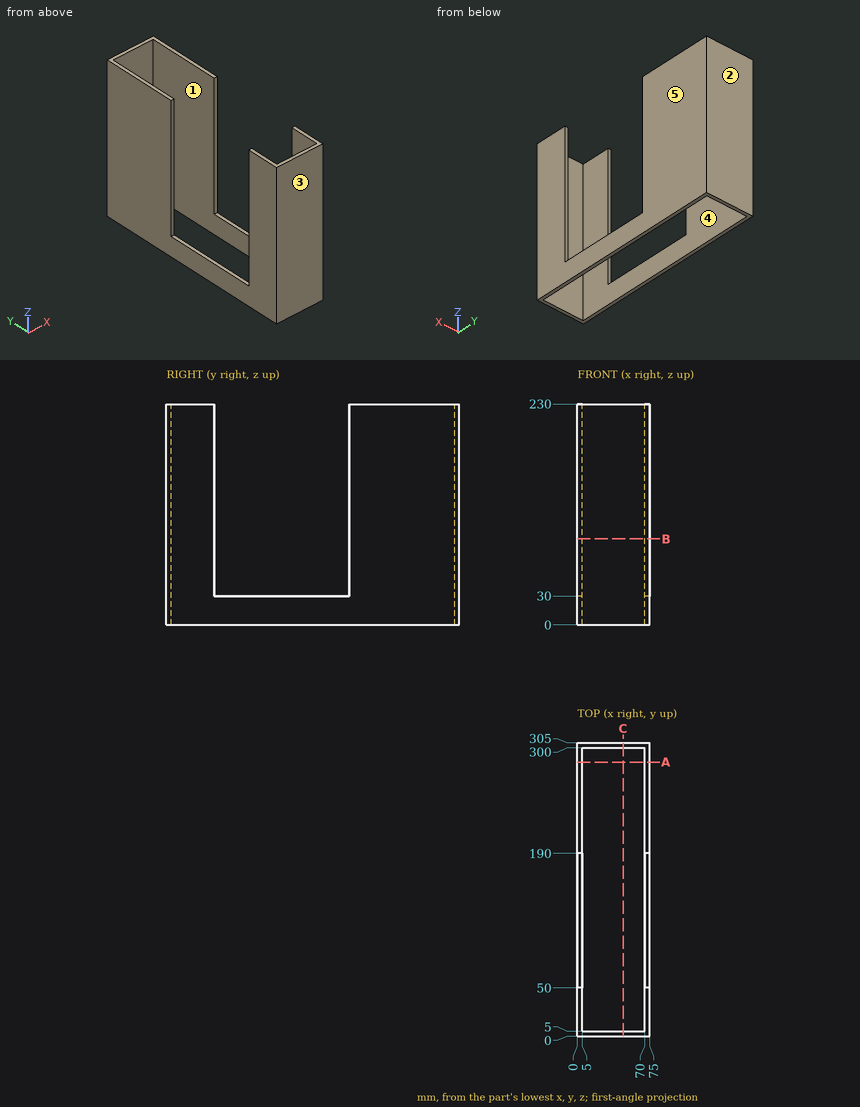
Study the drawing (mm; zero at the part's minimum x, y, z) and answer. A direction names the side the tool comes from. Coordinates: 2 decimals unless noted, no trailing zeros. Loops run counter-clockwise (first coordinate to the right, second up) from the corner with the lowest first, then second, coordinate; pieces in that order, holes last. Notation, with made-up numbers: M -33.5,46.5 L -29.5,46.5 A34 ccw -29.5,85.5 Z; hole C 35.5,73 d1. An arc over 180 degrees is marked long. Answer as a JSON object with one key per item and string values. Group by question number.
Item 1: This flat-tipped pin is pushed along its axis until it touches: P1, Ø2.5, axis at x = 73.5, y = 141, coming from the +Z side. Where does it stop, or does it pass through?
Item 2: Consider L1, parallel to X at y = 254.5, z = 208; L2, parallel to Y at x = 47, z = 215.5; L3, parallel to Y at x = 72, z = 149. Determine where each line is inside the solid, lowest interval first.
Item 3: Section A-A (y = 285) is taken. Write down the section's boundary in (x, z).
Item 4: Which of the six approach directions +Z, -Z, +X, -X, +Y, -Y give full straight-line access (tool end or side, diameter ignored) to the marked faces 1 and 2?
Item 5: Section C-C (x = 47.5) is taken. Write down the section's boundary in (y, z).
Item 6: Determine the mould class of the marked faces 3, 4 and 5 for opening direction Y: +Y half, -Y half, draft (parallel to the pull), parting line (faces both ways), or undercut.
Item 7: Section B-B (z = 89.5) is taken. Write down the section's boundary in (x, y), and give its area (3 significant figures).
Solved:
{
 "1": {"P1": "stops at z = 30"},
 "2": {"L1": "x = 0 to 5, 70 to 75", "L2": "y = 0 to 5, 300 to 305", "L3": "y = 0 to 50, 190 to 305"},
 "3": {"outline": "M 0,0 L 5,0 L 5,230 L 0,230 Z; M 70,0 L 75,0 L 75,230 L 70,230 Z"},
 "4": {"face 1": "+Z, -Z", "face 2": "+Z, -Z, +X, -X, +Y"},
 "5": {"outline": "M 0,0 L 5,0 L 5,230 L 0,230 Z; M 300,0 L 305,0 L 305,230 L 300,230 Z"},
 "6": {"face 3": "-Y half", "face 4": "undercut", "face 5": "draft"},
 "7": {"outline": "M 0,0 L 75,0 L 75,50 L 70,50 L 70,5 L 5,5 L 5,50 L 0,50 Z; M 0,190 L 5,190 L 5,300 L 70,300 L 70,190 L 75,190 L 75,305 L 0,305 Z", "area": "2,300 mm2"}
}
